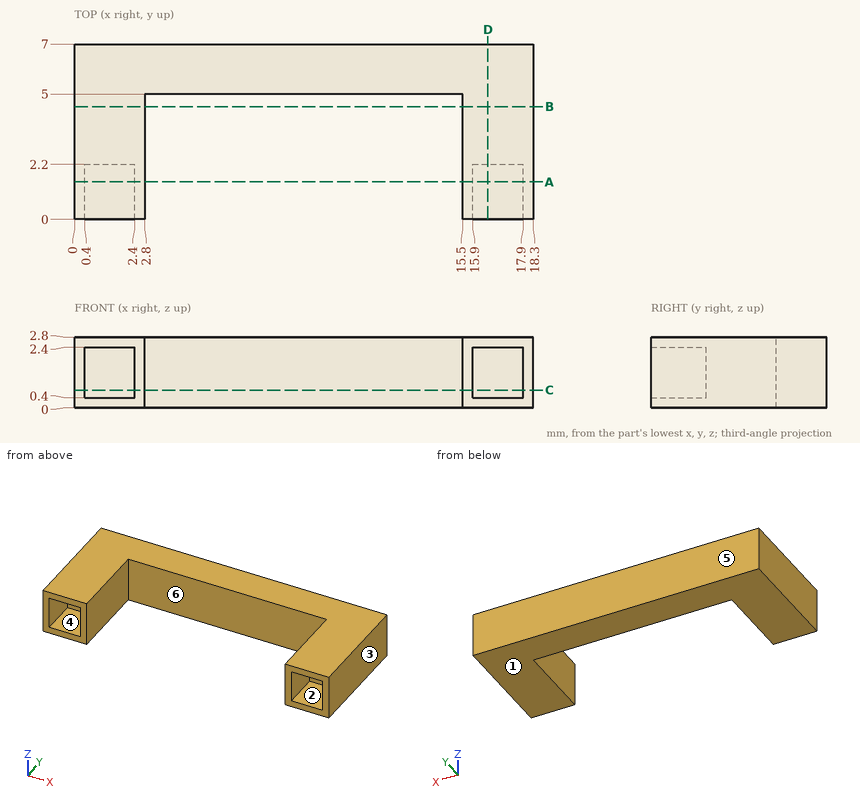
Check sheet for the drawn part. Datum: minimum x, y, z corner. Units: mm. A direction names the side the tool comes from. Round coordinates to 2 decimals unless told otherwise and drop trailing zeros. Order: outer loops, then holes, each group sorted by start corner. A loop starts at its lowest first (then second) coordinate and runs counter-clockwise, first axis right, second up. Notation, with made-up numbers: (64.25, 43) -> (73.25, 43) arc R24 cw to (73.25, 70) -> close; hole circle Ø8 at (56.25, -32.75). An arc over 180 degrees is marked (long way). Return JSON: item names as keys, results as strings. Group by question number.
Q1. Material ranges on probe 1 along X at (y, z) = (0.5, 1.6); probe 2 along X at (y, z) = (4.5, 2.1); probe 3 along Y at (x, z) = (9.75, 2.3), recorded low to high. Write a range as from..to.
Q2. Section check A-A, the plane y = 1.5. Record the boundary of the cut face in (x, z), plus the area to 3 significant figures.
Q3. Gauge pin test, flat end, axial feed: pin 1 (0.6 mm diameter, centred on x = 1, z = 2, fed in from -Y). Record the tip position at first contact, or that the pin passes through.
Q4. Section check C-C, the plane z = 0.7. Record the boundary of the cut face in (x, y), plus the area to 3 significant figures.
Q5. Release check for a two-part mould opening along X. For the marked faces 1, 2 and 3 record: released by +X, released by -X, zero draft, split by the parting line, or undercut.
Q6. Section check B-B, the plane y = 4.5. Record the boundary of the cut face in (x, z), plus the area to 3 significant figures.
Q7. Tool access check on the marked faces 4, 5 and 6. Record the directions out of +Z, -Z, +X, -X, +Y, -Y that give a thin tool (end or side, any length) a straight path to the whole face; none if there is none.
Q8. Section check D-D, the plane x = 16.5. Record the boundary of the cut face in (y, z), plus the area to 3 significant figures.
Numbers:
{
 "1": {"probe 1": "0..0.4, 2.4..2.8, 15.5..15.9, 17.9..18.3", "probe 2": "0..2.8, 15.5..18.3", "probe 3": "5..7"},
 "2": {"outline": "(0, 0) -> (2.8, 0) -> (2.8, 2.8) -> (0, 2.8) -> close; (15.5, 0) -> (18.3, 0) -> (18.3, 2.8) -> (15.5, 2.8) -> close; hole (0.4, 0.4) -> (2.4, 0.4) -> (2.4, 2.4) -> (0.4, 2.4) -> close; hole (15.9, 0.4) -> (17.9, 0.4) -> (17.9, 2.4) -> (15.9, 2.4) -> close", "area": "7.68 mm^2"},
 "3": {"pin 1": "y = 2.2"},
 "4": {"outline": "(0, 0) -> (0.4, 0) -> (0.4, 2.2) -> (2.4, 2.2) -> (2.4, 0) -> (2.8, 0) -> (2.8, 5) -> (15.5, 5) -> (15.5, 0) -> (15.9, 0) -> (15.9, 2.2) -> (17.9, 2.2) -> (17.9, 0) -> (18.3, 0) -> (18.3, 7) -> (0, 7) -> close", "area": "55.8 mm^2"},
 "5": {"face 1": "zero draft", "face 2": "undercut", "face 3": "released by +X"},
 "6": {"outline": "(0, 0) -> (2.8, 0) -> (2.8, 2.8) -> (0, 2.8) -> close; (15.5, 0) -> (18.3, 0) -> (18.3, 2.8) -> (15.5, 2.8) -> close", "area": "15.7 mm^2"},
 "7": {"face 4": "-Y", "face 5": "+Z, -Z, +X, -X, +Y", "face 6": "+Z, -Z, -Y"},
 "8": {"outline": "(0, 0) -> (7, 0) -> (7, 2.8) -> (0, 2.8) -> (0, 2.4) -> (2.2, 2.4) -> (2.2, 0.4) -> (0, 0.4) -> close", "area": "15.2 mm^2"}
}
